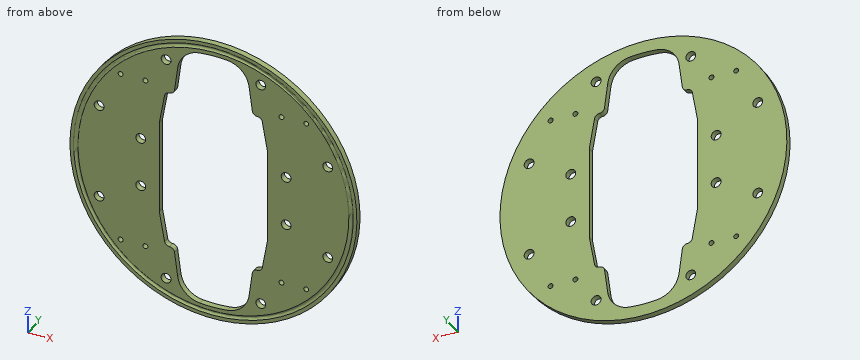
```python
from build123d import *

# Parameters (mm, degrees)
SKETCH1_R                      = 147.24126
BOSS_EXTRUDE1_DEPTH            = 6.35
F_3_8_CLEARANCE_HOLE1_D        = 10.0838
SKETCH6_R                      = 2.38125
F_3_8_CLEARANCE_HOLE2_D        = 10.0838
FILLET1_R                      = 5.08
F_7_0_201_DIAMETER_HOLE1_D     = 5.1054
F_7_0_201_DIAMETER_HOLE1_DEPTH = 6.35


with BuildPart() as part:
    # Sketch1 → Boss-Extrude1 (new body)
    with BuildSketch(Plane(origin=(0, 0, 0), x_dir=(1, 0, 0), z_dir=(0, 1, 0))):
        with Locations(Location((0, 0, 0), (0, 0, 270))):
            Circle(SKETCH1_R)
        with BuildLine():
            Line((-36.612699479, 112.267654933), (-40.525102973, 82.55))
            Line((-40.525102973, 82.55), (-49.404280199, 82.55))
            Line((-49.404280199, 82.55), (-55.5625, 47.625))
            Line((-55.5625, 47.625), (-55.5625, -47.625))
            Line((-55.5625, -47.625), (-49.404280199, -82.55))
            Line((-49.404280199, -82.55), (-40.525102973, -82.55))
            Line((-40.525102973, -82.55), (-36.612699479, -112.267654933))
            ThreePointArc((-36.612699479, -112.267654933), (-29.152114648, -127.148076316), (-14.080127521, -134.213659845))
            ThreePointArc((-14.080127521, -134.213659845), (0, -134.9502), (14.080127521, -134.213659845))
            ThreePointArc((14.080127521, -134.213659845), (29.152114648, -127.148076316), (36.612699479, -112.267654933))
            Line((36.612699479, -112.267654933), (40.525102973, -82.55))
            Line((40.525102973, -82.55), (49.404280199, -82.55))
            Line((49.404280199, -82.55), (55.5625, -47.625))
            Line((55.5625, -47.625), (55.5625, 47.625))
            Line((55.5625, 47.625), (49.404280199, 82.55))
            Line((49.404280199, 82.55), (40.525102973, 82.55))
            Line((40.525102973, 82.55), (36.612699479, 112.267654933))
            ThreePointArc((36.612699479, 112.267654933), (29.152114648, 127.148076316), (14.080127521, 134.213659845))
            ThreePointArc((14.080127521, 134.213659845), (0, 134.9502), (-14.080127521, 134.213659845))
            ThreePointArc((-14.080127521, 134.213659845), (-29.152114648, 127.148076316), (-36.612699479, 112.267654933))
        make_face(mode=Mode.SUBTRACT)
    extrude(amount=BOSS_EXTRUDE1_DEPTH)

    # 3/8 Clearance Hole1 (through all)
    with Locations(Plane(origin=(0, 6.35, 0), x_dir=(1, 0, 0), z_dir=(0, 1, 0))):
        with Locations((-117.332700629, 48.60079591), (-48.60079591, 117.332700629), (48.60079591, 117.332700629), (117.332700629, 48.60079591), (117.332700629, -48.60079591), (48.60079591, -117.332700629), (-48.60079591, -117.332700629), (-117.332700629, -48.60079591)):
            Hole(F_3_8_CLEARANCE_HOLE1_D / 2)

    # Sketch6 → Cut-Revolve1 (revolve, cut)
    with BuildSketch(Plane(origin=(0, 0, 0), x_dir=(0, 0, -1), z_dir=(1, 0, 0)), mode=Mode.PRIVATE) as cut_revolve1_sk:
        with Locations((141.2875, -0.79375)):
            Circle(SKETCH6_R)
    revolve(cut_revolve1_sk.sketch.rotate(Axis((0, 0, 0), (0, -1, 0)), 180), axis=Axis((0, 0, 0), (0, -1, 0)), mode=Mode.SUBTRACT)

    # 3/8 Clearance Hole2 (through all)
    with Locations(Plane(origin=(0, 0, 0), x_dir=(-1, 0, 0), z_dir=(0, -1, 0))):
        with Locations((74.6125, -25.4), (74.6125, 25.4), (-74.6125, 25.4), (-74.6125, -25.4)):
            Hole(F_3_8_CLEARANCE_HOLE2_D / 2)

    # Fillet1
    fillet1_edges = [part.edges().sort_by_distance(p)[0] for p in [
        (-40.525102973, 3.175, -82.55),
        (-49.404280199, 3.175, -82.55),
        (-55.5625, 3.175, -47.625),
        (-55.5625, 3.175, 47.625),
        (-49.404280199, 3.175, 82.55),
        (-40.525102973, 3.175, 82.55),
        (40.525102973, 3.175, 82.55),
        (49.404280199, 3.175, 82.55),
        (55.5625, 3.175, 47.625),
        (55.5625, 3.175, -47.625),
        (49.404280199, 3.175, -82.55),
        (40.525102973, 3.175, -82.55),
    ]]
    fillet(fillet1_edges, radius=FILLET1_R)

    # #7 (0.201) Diameter Hole1
    with Locations(Plane(origin=(0, 6.35, 0), x_dir=(1, 0, 0), z_dir=(0, 1, 0))):
        with Locations((-69.85, -88.9), (-95.25, -88.9), (-95.25, 88.9), (-69.85, 88.9), (0, 0), (69.85, 88.9), (95.25, 88.9), (95.25, -88.9), (69.85, -88.9)):
            Hole(F_7_0_201_DIAMETER_HOLE1_D / 2, depth=F_7_0_201_DIAMETER_HOLE1_DEPTH)


solid = part.part
```
The model under review builds one solid part; all positions refer to its coordinate system, in mm. Round coordinates to 2 decimals unless told otherwise and drop trailing zeros. Loops run counter-clockwise (first coordinate to the right, second up) from the corner with the lowest first, then second, coordinate; pieces in that order, holes last. Notation, with made-up numbers: (49.25, 62.5) -> (73.25, 62.5) arc R11 cw to (73.25, 69.5) -> close; hole circle Ø10 at (82.5, 79). An arc over 180 degrees is marked (long way). Answer as a JSON object with one key per item and string values. Group by question number.
1) For line 1 (Z direction, x = 95.25, y = 5); line 2 (X direction, y = 5.75, z = -91); line 3 (X direction, y = 3.75, z = -29), list the stretches that pass through material, from the lowest coordinate up. Write a range as [from, to].
2) We need section C-C on y = 2.75. Give the number of separate pieces and of enclosed holes in the cut face, then the cut area to 3 significant figures.
3) For pin 1 Ø6 at (x, z) = (74.61, -25.4) entering from -Y; pin 2 Ø1 at (y, z) = (1.5, -47) entering from +X; pin 3 Ø3 at (x, y) = (24, 1.5) entering from +Z; pin 4 Ø2 at (y, z) = (1, 30.5) entering from +X, all flat-tipped, find the tip position at first contact; note any pin that passes through.
4) We need section B-B on x = 0. Write out the cut boundary in (y, z).
5) We need section A-A on z = 0. Write out the cut boundary in (x, y), then the cut area to 3 significant figures.
Result set:
{
 "1": {"line 1": "[-112.28, -91.45], [-86.35, 86.35], [91.45, 112.28]", "line 2": "[-115.75, -96.7], [-93.8, -71.3], [-68.4, -39.41], [39.41, 68.4], [71.3, 93.8], [96.7, 115.75]", "line 3": "[-144.36, -78.14], [-71.08, -55.56], [55.56, 71.08], [78.14, 144.36]"},
 "2": {"separate pieces": "1", "enclosed holes": "21", "area": "41,800 mm²"},
 "3": {"pin 1": "through", "pin 2": "x = 139.71", "pin 3": "z = 145.51", "pin 4": "x = 144.26"},
 "4": {"outline": "(0, -147.24) -> (6.35, -147.24) -> (6.35, -134.95) -> (0, -134.95) -> (0, -139.04) arc R2.38 cw to (0, -143.53) -> close; (0, 134.95) -> (6.35, 134.95) -> (6.35, 147.24) -> (0, 147.24) -> (0, 143.53) arc R2.38 cw to (0, 139.04) -> close"},
 "5": {"outline": "(-147.24, 0) -> (-143.53, 0) arc R2.38 cw to (-139.04, 0) -> (-55.56, 0) -> (-55.56, 6.35) -> (-147.24, 6.35) -> close; (55.56, 0) -> (139.04, 0) arc R2.38 cw to (143.53, 0) -> (147.24, 0) -> (147.24, 6.35) -> (55.56, 6.35) -> close", "area": "1,150 mm²"}
}
